Source: CAD feature listing. Evaluate the final solid. Frame: model axes, mm. Face numbers are marked on the shaded views. A direction names the side the tool comes from. Round coordinates to 2 decimals unless told otherwise and drop trailing zeros. Write each loop counter-clockwise with the first axis right and the second up, starting at its lowest first coordinate (ties: lowest second). Pieces come first, ordered by that corner, then holes. Notation, with made-up numbers: M 19,68.5 L 40,68.5 A18 ccw 40,77.5 Z; hole C 19,88 d11. An arc over 180 degrees is marked long. Use a Markdown table: item, result.
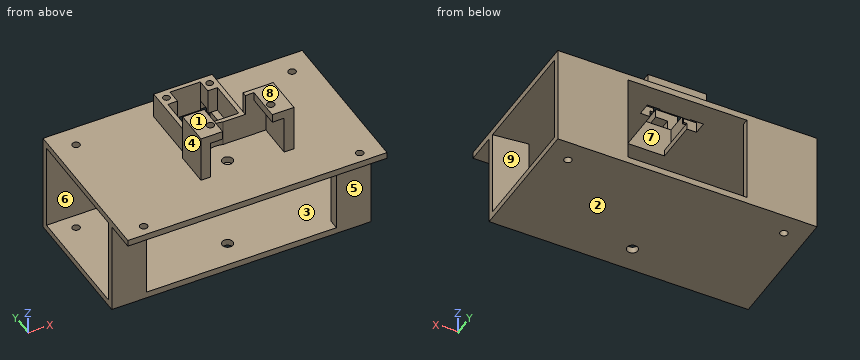
```python
from build123d import *
from build123d.topology import SkipClean

# Parameters (mm, degrees)
SKETCH_1_W           = 120
SKETCH_1_H           = 60
EXTRUDE_1_DEPTH      = 47
SHELL_2_T            = -3
SKETCH_2_W           = 55
SKETCH_2_H           = 41
CUT_EXTRUDE_1_DEPTH  = 3
SKETCH_5_W           = 88
SKETCH_5_H           = 41
CUT_EXTRUDE_3_DEPTH  = 10
SKETCH_6_R           = 2.5
CUT_EXTRUDE_4_DEPTH  = 82.908485519
EXTRUDE_4_REACH      = 82.225
CUT_EXTRUDE_5_REACH  = 83.908
SKETCH_9_W           = 17
SKETCH_9_H           = 25
SKETCH_10_W          = 27
SKETCH_10_H          = 29
SKETCH_10_R          = 1.6
EXTRUDE_5_DEPTH      = 12
SKETCH_14_W          = 10
SKETCH_14_H          = 16
SKETCH_14_R          = 1.75
EXTRUDE_7_DEPTH      = 22
SKETCH_15_R          = 10.5
CUT_EXTRUDE_7_DEPTH  = 12
CUT_EXTRUDE_8_DEPTH  = 6
CUT_EXTRUDE_9_REACH  = 83.908
SKETCH_19_W          = 34
SKETCH_19_H          = 16
SKETCH_16_W          = 14
SKETCH_16_H          = 2
EXTRUDE_8_DEPTH      = 22
SKETCH_20_W          = 6
SKETCH_20_H          = 6
CUT_EXTRUDE_10_DEPTH = 5
SKETCH_21_W          = 120
SKETCH_21_H          = 3
EXTRUDE_9_DEPTH      = 14
SKETCH_11_R          = 1.75
CUT_EXTRUDE_6_DEPTH  = 89.005681635


with BuildPart() as part:
    # 草图1 → 凸台-拉伸1 (new body)
    with BuildSketch(Plane(origin=(0, 0, 0), x_dir=(1, 0, 0), z_dir=(0, 0, -1))):
        Rectangle(SKETCH_1_W, SKETCH_1_H)
    extrude(amount=EXTRUDE_1_DEPTH)

    # 抽壳2
    shell_2_openings = [part.faces().sort_by_distance(p)[0] for p in [
        (60, 0, -23.5),
        (-60, 0, -23.5),
    ]]
    offset(amount=SHELL_2_T, openings=shell_2_openings, kind=Kind.INTERSECTION)

    # 草图2 → 切除-拉伸1 (cut)
    with BuildSketch(Plane(origin=(0, 30, 45), x_dir=(-1, 0, 0), z_dir=(0, -1, 0))):
        with Locations((0, 68.5)):
            Rectangle(SKETCH_2_W, SKETCH_2_H)
    extrude(amount=CUT_EXTRUDE_1_DEPTH, mode=Mode.SUBTRACT)

    # 草图5 → 切除-拉伸3 (cut)
    with BuildSketch(Plane.XZ.offset(30)):
        with Locations((0, -23.5)):
            Rectangle(SKETCH_5_W, SKETCH_5_H)
    extrude(amount=-CUT_EXTRUDE_3_DEPTH, mode=Mode.SUBTRACT)

    # 草图6 → 切除-拉伸4 (cut, through all)
    with BuildSketch(Plane.XY):
        with Locations((0, -18)):
            Circle(SKETCH_6_R)
    extrude(amount=-CUT_EXTRUDE_4_DEPTH, mode=Mode.SUBTRACT)

    # 草图8 → 凸台-拉伸4 (add, up to next)
    with BuildSketch(Plane(origin=(0, 0, -44), x_dir=(-1, 0, 0), z_dir=(0, 0, -1)), mode=Mode.PRIVATE) as extrude_4_sk1:
        Polygon((-60, -27), (-44, -25.270549885), (-44, -30), (-60, -30), align=None)
    extrude_4_tool1 = extrude(extrude_4_sk1.sketch, amount=-EXTRUDE_4_REACH, mode=Mode.PRIVATE) - part.part
    extrude_4 = extrude_4_tool1.solids().sort_by_distance((51.403338, -28.035391, -44))[0]
    add(extrude_4)

    # 镜向1: 凸台-拉伸4 across plane
    add(extrude_4.mirror(Plane(origin=(0, 0, 0), x_dir=(0, 0, 1), z_dir=(1, 0, 0))))

    # 草图9 → 切除-拉伸5 (cut, up to next)
    with BuildSketch(Plane.XY, mode=Mode.PRIVATE) as cut_extrude_5_sk1:
        with Locations((0, 6.5)):
            Rectangle(SKETCH_9_W, SKETCH_9_H)
    cut_extrude_5_tool1 = extrude(cut_extrude_5_sk1.sketch, amount=-CUT_EXTRUDE_5_REACH, mode=Mode.PRIVATE) & part.part
    add(cut_extrude_5_tool1.solids().sort_by_distance((0, 6.5, 0))[0], mode=Mode.SUBTRACT)

    # 草图10 → 凸台-拉伸5 (add)
    with BuildSketch(Plane.XY):
        with Locations((0, 6.5)):
            Rectangle(SKETCH_10_W, SKETCH_10_H)
        with Locations(Location((-10, 16.5, 0), (0, 0, 339.635865194))):
            Circle(SKETCH_10_R, mode=Mode.SUBTRACT)
        with Locations(Location((10, 16.5, 0), (0, 0, 159.635865194))):
            Circle(SKETCH_10_R, mode=Mode.SUBTRACT)
        Polygon((-11.5, -6), (11.5, -6), (11.5, 12.5), (7, 12.5), (7, 19), (-7, 19), (-7, 12.5), (-11.5, 12.5), align=None, mode=Mode.SUBTRACT)
    extrude(amount=EXTRUDE_5_DEPTH)

    # 草图14 → 凸台-拉伸7 (add)
    # profile 1 of 2: a face of its own
    with BuildSketch(Plane.XY):
        with Locations((-10.5, -16)):
            Rectangle(SKETCH_14_W, SKETCH_14_H)
        with Locations((-8, -18)):
            Circle(SKETCH_14_R, mode=Mode.SUBTRACT)
    # profile 2 of 2: a face of its own
    with BuildSketch(Plane.XY):
        with Locations((22.5, -16)):
            Rectangle(SKETCH_14_W, SKETCH_14_H)
        with Locations((20, -18)):
            Circle(SKETCH_14_R, mode=Mode.SUBTRACT)
    extrude(amount=EXTRUDE_7_DEPTH)

    # 草图15 → 切除-拉伸7 (cut)
    with BuildSketch(Plane.XY):
        with Locations((0, -18)):
            Circle(SKETCH_15_R)
    extrude(amount=CUT_EXTRUDE_7_DEPTH, mode=Mode.SUBTRACT)

    # 草图17 → 切除-拉伸8 (cut)
    with SkipClean():  # the faces are left unmerged after this step: merging them gives an invalid solid
        with BuildSketch(Plane(origin=(0, 0, 12), x_dir=(-1, 0, 0), z_dir=(0, 0, -1))):
            with BuildLine():
                Line((5.5, -9.05572809), (5.5, -24))
                Line((5.5, -24), (8.61684397, -24))
                ThreePointArc((8.61684397, -24), (10.278819808, -15.856203519), (5.5, -9.05572809))
            make_face()
        extrude(amount=-CUT_EXTRUDE_8_DEPTH, mode=Mode.SUBTRACT)

    # 切除-拉伸9: up to this face of the body (flat: up to its plane)
    cut_extrude_9_end = Plane(part.part.faces().sort_by_distance((-5.657585298, -16.527864045, 18))[0])
    # 草图19 → 切除-拉伸9 (cut, up to the picked face)
    with BuildSketch(Plane.XY, mode=Mode.PRIVATE) as cut_extrude_9_sk1:
        with Locations((6, -16)):
            Rectangle(SKETCH_19_W, SKETCH_19_H)
    cut_extrude_9_tool1 = split(extrude(cut_extrude_9_sk1.sketch, amount=CUT_EXTRUDE_9_REACH, mode=Mode.PRIVATE), bisect_by=cut_extrude_9_end, keep=Keep.BOTH, mode=Mode.PRIVATE)
    add(cut_extrude_9_tool1.solids().sort_by(Axis((6, -16, 0), (0, 0, 1)))[0], mode=Mode.SUBTRACT)

    # 草图16 → 凸台-拉伸8 (add)
    with BuildSketch(Plane.XY):
        with Locations((20.5, -7)):
            Rectangle(SKETCH_16_W, SKETCH_16_H)
    extrude(amount=EXTRUDE_8_DEPTH)

    # 草图20 → 切除-拉伸10 (cut)
    with BuildSketch(Plane(origin=(0, 0, -3), x_dir=(-1, 0, 0), z_dir=(0, 0, -1))):
        with Locations((-10, 16.5)):
            Rectangle(SKETCH_20_W, SKETCH_20_H)
        with Locations((10, 16.5)):
            Rectangle(SKETCH_20_W, SKETCH_20_H)
    extrude(amount=-CUT_EXTRUDE_10_DEPTH, mode=Mode.SUBTRACT)

    # 草图21 → 凸台-拉伸9 (add)
    with BuildSketch(Plane.XZ.offset(30)):
        with Locations((0, -1.5)):
            Rectangle(SKETCH_21_W, SKETCH_21_H)
    extrude(amount=EXTRUDE_9_DEPTH)

    # 草图11 → 切除-拉伸6 (cut, through all)
    with BuildSketch(Plane(origin=(0, 0, 0), x_dir=(-1, 0, 0), z_dir=(0, 0, -1))):
        with Locations(Location((-50, 20, 0), (0, 0, 180))):
            Circle(SKETCH_11_R)
        with Locations(Location((50, 20, 0), (0, 0, 180))):
            Circle(SKETCH_11_R)
        with Locations(Location((-50, -39, 0), (0, 0, 180))):
            Circle(SKETCH_11_R)
        with Locations(Location((50, -39, 0), (0, 0, 180))):
            Circle(SKETCH_11_R)
    extrude(amount=CUT_EXTRUDE_6_DEPTH, mode=Mode.SUBTRACT)


solid = part.part
```
Q1. Section B-B on x = 20. Return loops of the section in (y, z).
Results are:
| item | result |
|---|---|
| outline | M -44,-3 L 30,-3 L 30,0 L -6,0 L -6,22 L -16.25,22 L -16.25,18 L -8,18 L -8,0 L -44,0 Z; M -30,-47 L 30,-47 L 30,-44 L -30,-44 Z; M -24,18 L -19.75,18 L -19.75,22 L -24,22 Z |
Q2. Mould query, pull axis Z, two halves, no side actions, for the marked faces 1, 2, 3 and 4. Classes: +Z half, -Z half, draft (parallel to the pull), parting line (faces both ways), or undercut.
Results are:
| item | result |
|---|---|
| face 1 | +Z half |
| face 2 | -Z half |
| face 3 | undercut |
| face 4 | draft |
Q3. Section D-D on z = 15.5. Return loops of the section in (x, y).
Results are:
| item | result |
|---|---|
| outline | M -15.5,-24 L -11,-24 L -11,-8 L -15.5,-8 Z; M 13.5,-8 L 23,-8 L 23,-24 L 27.5,-24 L 27.5,-6 L 13.5,-6 Z |
Q4. Section A-A on z = -23. Return loops of the section in (x, y), plus the area to 3 significant figures.
Results are:
| item | result |
|---|---|
| outline | M -60,-30 L -44,-30 L -44,-25.27 L -60,-27 Z; M -60,27 L -27.5,27 L -27.5,30 L -60,30 Z; M 27.5,27 L 60,27 L 60,30 L 27.5,30 Z; M 44,-30 L 60,-30 L 60,-27 L 44,-25.27 Z |
| area | 319 mm^2 |
Q5. First-contact query: pin 1 Ø1.3 at (x, z) = (-10.5, 8.5) entering from -Y; pin 2 Ø4 at (x, y) = (-30.5, -33.5) entering from -Z; pin 3 Ø7.5 at (x, z) = (-5, 5.5) entering from +Y. Flat tips, straight axial feed; report the tip coordinate or a pass-through.
Results are:
| item | result |
|---|---|
| pin 1 | y = -24 |
| pin 2 | z = -3 |
| pin 3 | y = 21 |
Q6. Reachability of the marked faces 5, 6, 7, 8 and 9 from +Z, -Z, +X, -X, +Y, -Y: full face, straight path, thin tool, end or side. Return the list, or none.
Results are:
| item | result |
|---|---|
| face 5 | -Z, +X, -X, -Y |
| face 6 | +X, -X |
| face 7 | +Z |
| face 8 | +Z, +X, -X, +Y, -Y |
| face 9 | +X |
Q7. Section C-C on y = 3. Return loops of the section in (x, z), plus the area to 3 significant figures.
Results are:
| item | result |
|---|---|
| outline | M -60,-47 L 60,-47 L 60,-44 L -60,-44 Z; M -60,-3 L -8.5,-3 L -8.5,0 L -11.5,0 L -11.5,12 L -13.5,12 L -13.5,0 L -60,0 Z; M 8.5,-3 L 60,-3 L 60,0 L 13.5,0 L 13.5,12 L 11.5,12 L 11.5,0 L 8.5,0 Z |
| area | 717 mm^2 |
Q8. Line query: L1, parallel to X at y = -18, z = 19; L2, parallel to Y at x = 50, z = -0.65; L3, parallel to Y at x = -10, z = 7. Output: solid intervals per line, ascending.
Results are:
| item | result |
|---|---|
| L1 | -15.5 to -9.75, -6.25 to -5.5, 17.5 to 18.25, 21.75 to 27.5 |
| L2 | -44 to -40.75, -37.25 to 18.25, 21.75 to 30 |
| L3 | -8 to -6, 12.5 to 14.9, 18.1 to 21 |
